Build history of the part. All positions in model axes, mm. A direction names the side the tool comes from. Give positions to 0.01 mm unless a question says otherwise; leave off trailing zeros. Write each loop counter-clockwise with the first axis right and the second up, starting at its lowest first coordinate (ties: lowest second). Pieces come first, ordered by that corner, then holes. Notation, with made-up numbers: (4.5, 25.5) -> (20.5, 25.5) arc R19 ccw to (20.5, 38.5) -> close; hole circle Ø4 at (0.25, -21.75). An arc over 180 degrees is marked (long way). One line per question, with ' | ' between items. Start each with the question number.
(1) Pin check, flat tips, straight feed: P1, Ø8, axis at x = 6.5, z = 20.5, coming from the +Y side; P2, Ø1, axis at y = -9.5, z = 17.5, coming from the +X side; P3, Ø5, axis at y = -6.5, z = -4, coming from the +X side. Stop position of each tip, or through.
(2) Pull direction X, two halves, no side cores. Call faces 1 (the flat face through (-8.3, -6.3, 18.3)), 2 (the flat face through (-9, -12.7, 17)), 3 (the flat face through (-10, -10, -5.475)): released by +X, released by -X, zero draft, split by the parting line, or undercut.
(3) Band-saw the part on A-A, the plane y = -9.5. Give the cut face in (x, z) (1 decimal).
(4) Drill centre lines: probe 1 along X at (y, z) = (-8, -9); probe 2 along X at (y, z) = (-9, 7); probe 3 along Z at (x, y) = (-12, -11.25) (3 decimals). Where is each one in solid material? Low to high. Write a range as from..to.
(5) Band-saw the part on B-B, the plane z = -9.5. Give the cut face in (x, y).
(6) Tool access for faces 4 (the flat face through (8.06, -4.85, 16.04)), 5 (the flat face through (0, -6, -8)), 6 (the cylindrical face through (-10.14, -6.35, -10.3)): list every direction of +Z, -Z, +X, -X, +Y, -Y with a clear straight run to the whole face (end or side of a thin tool).
(7) Band-saw the part on C-C, the plane y = -3.5. Give the cut face in (x, z).
from build123d import *

# Parameters (mm, degrees)
F1_DEPTH = 12.7
F2_R     = 6.35
F3_DEPTH = 39.8215080757
F4_R     = 6.35
F5_DEPTH = 9.525


with BuildPart() as f1:
    # F0 (on Front) → F1 (new body)
    with BuildSketch(Plane.XZ):
        Polygon((-20, 11.5470053838), (-20, -15), (0, -15), (0, 0), (12.9903810568, 7.5), (2.9903810568, 24.8205080757), align=None)
    extrude(amount=F1_DEPTH)

    # F2 (on face) → F3 (cut, through all)
    with BuildSketch(Plane(origin=(12.9903810568, 0, 7.5), x_dir=(0, 1, 0), z_dir=(0.8660254038, 0, 0.5))):
        with Locations((-12.7, 10)):
            Circle(F2_R)
    extrude(amount=-F3_DEPTH, mode=Mode.SUBTRACT)

    # F4 (on face) → F5 (cut)
    with BuildSketch(Plane(origin=(0, 0, -15), x_dir=(1, 0, 0), z_dir=(0, 0, -1))):
        with Locations((-10, 12.7)):
            Circle(F4_R)
    extrude(amount=-F5_DEPTH, mode=Mode.SUBTRACT)


solid = f1.part
Results:
1) P1: stops at y = 0 | P2: stops at x = 0.41 | P3: stops at x = 0
2) face 1: released by -X | face 2: zero draft | face 3: undercut
3) outline: (-20, -15) -> (-15.5, -15) -> (-15.5, -5.5) -> (-4.5, -5.5) -> (-4.5, -15) -> (0, -15) -> (0, 0) -> (13, 7.5) -> (10.7, 11.4) -> (-20, -6.3) -> close; (-20, 6.3) -> (5.2, 20.9) -> (3, 24.8) -> (-20, 11.5) -> close
4) probe 1: x = -20..-14.27, -5.73..0 | probe 2: x = -20..-18.2, 2.45..12.12 | probe 3: z = -5.475..-2.52, 11.757..16.166
5) outline: (-20, -12.7) -> (-16.35, -12.7) arc R6.35 cw to (-3.65, -12.7) -> (0, -12.7) -> (0, 0) -> (-20, 0) -> close
6) face 4: +Z, +X, +Y, -Y | face 5: -Z, +X, +Y, -Y | face 6: -Z, -Y
7) outline: (-20, -15) -> (0, -15) -> (0, 0) -> (12.99, 7.5) -> (2.99, 24.82) -> (-20, 11.55) -> close
